Can you work these out from the model? Positions are in its coordinate system, mm. Face numbers are marked on the shaded views. A direction names the side the tool comes from. Coordinates: 2 decimals unless noted, no trailing zeros. Answer as CSV lines item,"result". Start each with the question number.
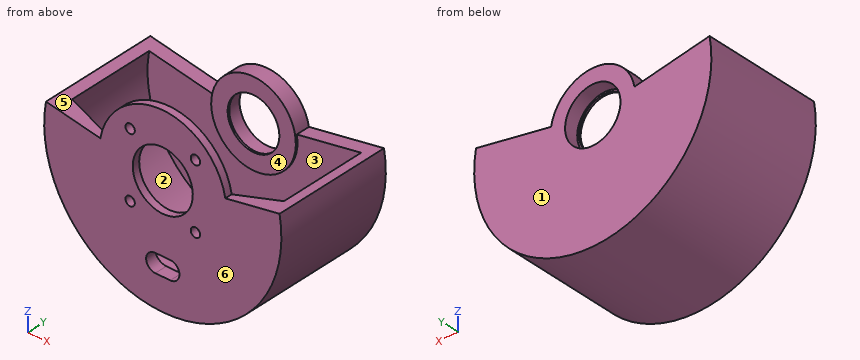
```python
from build123d import *

# Parameters (mm, degrees)
BOSS_EXTRUDE1_START = -14.125
SKETCH2_R           = 27.5
SKETCH2_R_2         = 13.000000035
SKETCH2_R_3         = 2.025
BOSS_EXTRUDE1_DEPTH = 3.175
BOSS_EXTRUDE2_START = 28.4275
SKETCH3_R           = 18.35
SKETCH3_R_2         = 12
BOSS_EXTRUDE2_DEPTH = 6
REVOLVE1_ANGLE      = 200
BOSS_EXTRUDE3_START = 0.79375
SKETCH5_R           = 18.35
SKETCH5_R_2         = 11.20625
BOSS_EXTRUDE3_DEPTH = 0.79375
CUT_EXTRUDE1_REACH  = 91.201


with BuildPart() as part:
    # Sketch2 → Boss-Extrude1 (new body)
    with BuildSketch(Plane(origin=(0, 0, 0), x_dir=(1, 0, 0), z_dir=(0, 1, 0)).offset(BOSS_EXTRUDE1_START)):
        with Locations(Location((0, 0, 0), (0, 0, 270))):
            Circle(SKETCH2_R)
        with Locations(Location((0, 0, 0), (0, 0, 270))):
            Circle(SKETCH2_R_2, mode=Mode.SUBTRACT)
        with Locations(Location((-14.142135624, -14.142135624, 0), (0, 0, 270))):
            Circle(SKETCH2_R_3, mode=Mode.SUBTRACT)
        with Locations(Location((14.142135624, -14.142135624, 0), (0, 0, 270))):
            Circle(SKETCH2_R_3, mode=Mode.SUBTRACT)
        with Locations(Location((14.142135624, 14.142135624, 0), (0, 0, 270))):
            Circle(SKETCH2_R_3, mode=Mode.SUBTRACT)
        with Locations(Location((-14.142135624, 14.142135624, 0), (0, 0, 270))):
            Circle(SKETCH2_R_3, mode=Mode.SUBTRACT)
    extrude(amount=-BOSS_EXTRUDE1_DEPTH)



with BuildPart() as body_2:
    # Sketch3 → Boss-Extrude2 (new body)
    with BuildSketch(Plane(origin=(0, 0, 0), x_dir=(1, 0, 0), z_dir=(0, 1, 0)).offset(BOSS_EXTRUDE2_START)):
        with Locations(Location((0, 0, 0), (0, 0, 270))):
            Circle(SKETCH3_R)
        with Locations(Location((0, 0, 0), (0, 0, 270))):
            Circle(SKETCH3_R_2, mode=Mode.SUBTRACT)
    extrude(amount=BOSS_EXTRUDE2_DEPTH)


with BuildPart() as part_1:
    add(part.part)

    add(body_2.part)  # Revolve1 merges body 2
    # Sketch4 → Revolve1 (revolve, symmetric)
    with BuildSketch(Plane(origin=(0, 0, 0), x_dir=(0, 0, -1), z_dir=(1, 0, 0))) as revolve1_sk:
        Polygon((27.5, -17.3), (51.38625, -17.3), (51.38625, 34.42749997), (18.35, 34.42749997), (18.35, 28.427500017), (46.62375, 28.427500017), (46.62375, -9.795291189), (27.5, -14.125), align=None)
    revolve(axis=Axis((0, -14.125, 0), (0, 1, 0)), revolution_arc=REVOLVE1_ANGLE / 2)
    revolve(revolve1_sk.sketch, axis=Axis((0, -14.125, 0), (0, -1, 0)), revolution_arc=REVOLVE1_ANGLE / 2)

    # Sketch5 → Boss-Extrude3 (add)
    with BuildSketch(Plane.XZ.offset(-28.427500017).offset(BOSS_EXTRUDE3_START)):
        with Locations(Location((0, 0, 0), (0, 0, 270))):
            Circle(SKETCH5_R)
        with Locations(Location((0, 0, 0), (0, 0, 270))):
            Circle(SKETCH5_R_2, mode=Mode.SUBTRACT)
    extrude(amount=-BOSS_EXTRUDE3_DEPTH)

    # Cut-Extrude1: up to this cone (the profile starts outside it)
    cut_extrude1_end = Plane(origin=(0, -17.3, 0), z_dir=(0, 1, 0)).offset(-3.051131024) * Cone(4.417e-06, 478.031284628, 108.228576807, align=(Align.CENTER, Align.CENTER, Align.MIN), mode=Mode.PRIVATE)
    # Sketch6 → Cut-Extrude1 (cut, up to the surface)
    with BuildSketch(Plane(origin=(0, -17.3, 0), x_dir=(-1, 0, 0), z_dir=(0, -1, 0)), mode=Mode.PRIVATE) as cut_extrude1_sk1:
        with BuildLine():
            Line((3.25, 29.61125), (-3.25, 29.61125))
            ThreePointArc((-3.25, 29.61125), (-7.21875, 33.58), (-3.25, 37.54875))
            Line((-3.25, 37.54875), (3.25, 37.54875))
            ThreePointArc((3.25, 37.54875), (7.21875, 33.58), (3.25, 29.61125))
        make_face()
    cut_extrude1_tool1 = extrude(cut_extrude1_sk1.sketch, amount=-CUT_EXTRUDE1_REACH, mode=Mode.PRIVATE) - cut_extrude1_end
    add(cut_extrude1_tool1.solids().sort_by_distance((0, -17.3, -33.58))[0], mode=Mode.SUBTRACT)


solid = part_1.part
```
Q1. Imagine slicing it at B-B (x = 0). State how many separate pieces and enclosed holes the cut face has, then the cut area to 3 significant figures.
Q2. For pin 1 (4 mm diameter, centred on y = -6.5, z = -9.5, fed in from -X); pin 2 (1.5 mm diameter, centred on y = -5, z = -38, fed in from -X); pin 3 (2.5 mm diameter, centred on x = 1.5, y = -15.5, fed in from +Z), each with a flat end and sliding along its axis, tell me the tip position at first contact or that it passes through.
Q3. If we mould it in two halves opening along Y, with no side actions, what happens to the marked faces 3, 4, 5 and 6? For each: released by +Y, released by -Y, zero draft, split by the parting line, or undercut.
Q4. Which directions (+Z, -Z, +X, -X, +Y, -Y) give clear straight access to the entire face, cutting with the end or side of a thin tool? Please do the marked faces 1 and 2.
Q5. I need wall thicknesses on L1, parallel to Y at x = 7.5, z = -23 (1 decimal); L2, parallel to X at y = 28.35, z = 0; L3, parallel to X at y = 5, z = 0. Which ranges of each line are inside material? Lowest first, please.
Entries:
1,separate pieces,"4"
1,enclosed holes,"0"
1,area,"662 mm2"
2,pin 1,"x = -50.84"
2,pin 2,"x = -35.4"
2,pin 3,"z = 27.5"
3,face 3,"undercut"
3,face 4,"undercut"
3,face 5,"zero draft"
3,face 6,"released by -Y"
4,face 1,"+Z, -Z, +X, -X, +Y"
4,face 2,"none"
5,L1,"-17.3 to -14.1, 28.4 to 34.4"
5,L2,"-51.39 to -46.62, -18.35 to -11.21, 11.21 to 18.35, 46.62 to 51.39"
5,L3,"-51.39 to -46.62, 46.62 to 51.39"
